Check sheet for the modelled part. Datum: model origin and axes. Units: mm. A direction names the side the tool comes from. Give positions to 0.01 mm unless a question says otherwise; leave off trailing zeros. Order: outer loops, then holes, each group sorted by start corner. A loop starts at its lowest first (then second) coordinate and runs counter-clockwise, first axis right, second up. Notation, with made-up numbers: (-26.5, -29) -> (-1.5, -29) arc R30 ccw to (-1.5, -1) -> close; hole circle Ø2 at (36, -26.5). An arc over 180 degrees is marked (long way). One line per question, with ' | ' between items.
Solid Edge part; units mm, degrees
sketch "Sketch1" plane through (0, 0, 0) normal (0, -1, 0) x (1, 0, 0)
  line L0 (10.16, 12.7) -> (-10.16, 12.7)
  arc A0 (-10.16, 12.7) -> (-12.7, 10.16) centre (-10.16, 10.16) ccw
  line L1 (-12.7, 10.16) -> (-12.7, -10.16)
  arc A1 (-12.7, -10.16) -> (-10.16, -12.7) centre (-10.16, -10.16) ccw
  line L2 (-10.16, -12.7) -> (10.16, -12.7)
  arc A2 (10.16, -12.7) -> (12.7, -10.16) centre (10.16, -10.16) ccw
  line L3 (12.7, -10.16) -> (12.7, 10.16)
  arc A3 (12.7, 10.16) -> (10.16, 12.7) centre (10.16, 10.16) ccw
extrude "Protrusion1" add sketch "Sketch1" against normal blind 1.5875
sketch "Sketch2" plane through (0, 0, 0) normal (0, -1, 0) x (1, 0, 0)
  circle A0 centre (-9.1186, 9.1186) radius 1.5875
  circle A1 centre (9.1186, 9.1186) radius 1.5875
  circle A2 centre (9.1186, -9.1186) radius 1.5875
  circle A3 centre (-9.1186, -9.1186) radius 1.5875
extrude "Cutout1" cut sketch "Sketch2" against normal through all
sketch "Sketch3" plane through (0, 0, 0) normal (0, -1, 0) x (1, 0, 0)
  circle A0 centre (0, 0) radius 7.874
extrude "ExtrudedProtrusion_2" add sketch "Sketch3" against normal blind 15.875 and the other way blind 3.175
sketch "Sketch4" plane through (0, 15.875, 0) normal (0, 1, 0) x (1, 0, 0)
  circle A0 centre (0, 0) radius 1.3843
extrude "ExtrudedProtrusion_3" add sketch "Sketch4" against normal blind 26.9748
Q1. Depth check by flat-ended pin: pin 1 Ø12.5 at (x, z) = (2, -1) entering from -Y; pin 2 Ø2 at (y, z) = (4, -6) entering from +X; pin 3 Ø3 at (y, z) = (4.5, -3.5) entering from -X; pin 4 Ø3 at (y, z) = (13, 7) entering from -X. Enter the tip coordinate at first touch or a pass-through.
Result sheet:
pin 1: stops at y = -11.1 | pin 2: stops at x = 6.08 | pin 3: stops at x = -7.62 | pin 4: stops at x = -5.63
Q2. Section check B-B (x = -8.75). Enter the section's corners in (y, z), and give its area (3 significant figures).
Result sheet:
outline: (0, -12.7) -> (1.59, -12.7) -> (1.59, -10.66) -> (0, -10.66) -> close; (0, -7.57) -> (1.59, -7.57) -> (1.59, 7.57) -> (0, 7.57) -> close; (0, 10.66) -> (1.59, 10.66) -> (1.59, 12.7) -> (0, 12.7) -> close | area: 30.5 mm2
Q3. Section check C-C (x = 0). Enter the section's corners in (y, z) (1 decimal), and give its area (3 significant figures).
Result sheet:
outline: (-11.1, -1.4) -> (-3.2, -1.4) -> (-3.2, -7.9) -> (0, -7.9) -> (0, -12.7) -> (1.6, -12.7) -> (1.6, -7.9) -> (15.9, -7.9) -> (15.9, 7.9) -> (1.6, 7.9) -> (1.6, 12.7) -> (0, 12.7) -> (0, 7.9) -> (-3.2, 7.9) -> (-3.2, 1.4) -> (-11.1, 1.4) -> close | area: 337 mm2
Q4. Mould release check, pull along Z, two halves, no side actions. Record for faces 1 (the face through (8.774, 0.783, -10.668)), 2 (the face through (-1.707, 8.631, -7.687)), 3 (the face through (-9.33, 0.78, 10.69)), 4 (the face through (12.7, 1, 0)): pulls with the +Z half, pulls with the -Z half, needs draft (parallel to the pull), parting line crosses it, or undercut.
Result sheet:
face 1: undercut | face 2: parting line crosses it | face 3: undercut | face 4: needs draft
Q5. Section check D-D (z = 0). Enter the section's corners in (x, y) (1 decimal), and give its area (3 significant figures).
Result sheet:
outline: (-12.7, 0) -> (-7.9, 0) -> (-7.9, -3.2) -> (-1.4, -3.2) -> (-1.4, -11.1) -> (1.4, -11.1) -> (1.4, -3.2) -> (7.9, -3.2) -> (7.9, 0) -> (12.7, 0) -> (12.7, 1.6) -> (7.9, 1.6) -> (7.9, 15.9) -> (-7.9, 15.9) -> (-7.9, 1.6) -> (-12.7, 1.6) -> close | area: 337 mm2
Q6. Access from +Z, -Z, +X, -X, +Y, -Y to the whole of each face (thin tool, end or side, straight path). Record for faces 5 (the face through (6, 1.588, 6)), 6 (the face through (11.976, 0.783, 11.936)), 7 (the face through (6, 0, 6)).
Result sheet:
face 5: +Y | face 6: +Z, +X, +Y, -Y | face 7: -Y
Q7. Thickness scan on line 1 (Y direction, x = 4.75, z = 4) (3 decimals); line 2 (Y direction, x = 11, z = -6.5); line 3 (Z direction, x = -0.25, y = 10.5). Record the ranges inside material, lowest first.
Result sheet:
line 1: y = -3.175 to 15.875 | line 2: y = 0 to 1.59 | line 3: z = -7.87 to 7.87
Q8. Section check A-A (z = 8.5). Enter the section's corners in (x, y).
Result sheet:
outline: (-12.7, 0) -> (-10.58, 0) -> (-10.58, 1.59) -> (-12.7, 1.59) -> close; (-7.66, 0) -> (7.66, 0) -> (7.66, 1.59) -> (-7.66, 1.59) -> close; (10.58, 0) -> (12.7, 0) -> (12.7, 1.59) -> (10.58, 1.59) -> close
